```python
from build123d import *

# Parameters (mm, degrees)
SKETCH1_W               = 20.4
SKETCH1_H               = 17.7
SKETCH1_W_2             = 14.4
SKETCH1_H_2             = 11.7
SKETCH1_R               = 3.15
BOSS_EXTRUDE1_DEPTH     = 25
SKETCH1_3_W             = 20.4
SKETCH1_3_H             = 17.7
SKETCH1_3_W_2           = 14.4
SKETCH1_3_H_2           = 11.7
BOSS_EXTRUDE2_DEPTH     = 30
SKETCH2_W               = 22.449827962
SKETCH2_H               = 3
CUT_EXTRUDE1_DEPTH      = 15
FILLET1_R               = 10
SKETCH3_W               = 50
SKETCH3_H               = 20
SKETCH3_R               = 3.15
BOSS_EXTRUDE3_DEPTH     = 3
SKETCH4_R               = 1.7
CUT_EXTRUDE2_DEPTH      = 39.13135193
BOSS_EXTRUDE4_DEPTH     = 3
BOSS_EXTRUDE5_DEPTH     = 3
CHAMFER1_SIZE           = 3
CHAMFER2_SIZE           = 1
FILLET3_R               = 2
SKETCH7_W               = 14.4
SKETCH7_H               = 3
CUT_EXTRUDE3_DEPTH      = 5
BOSS_EXTRUDE6_DEPTH     = 5
CUT_EXTRUDE4_DEPTH      = 38.132499243
CUT_EXTRUDE4_DEPTH_BACK = 38.132499243
BOSS_EXTRUDE7_DEPTH     = 20.4


with BuildPart() as part:
    # Sketch1 → Boss-Extrude1 (new body)
    # profile 1 of 2: a face of its own
    with BuildSketch(Plane(origin=(0, 0, 0), x_dir=(1, 0, 0), z_dir=(0, 1, 0))):
        Rectangle(SKETCH1_W, SKETCH1_H)
        Rectangle(SKETCH1_W_2, SKETCH1_H_2, mode=Mode.SUBTRACT)
    # profile 2 of 2: a face of its own
    with BuildSketch(Plane(origin=(0, 0, 0), x_dir=(1, 0, 0), z_dir=(0, 1, 0))):
        Rectangle(SKETCH1_W_2, SKETCH1_H_2)
        with Locations(Location((0, 0, 0), (0, 0, 270))):
            Circle(SKETCH1_R, mode=Mode.SUBTRACT)
    extrude(amount=BOSS_EXTRUDE1_DEPTH)

    # Sketch1<3> → Boss-Extrude2 (add)
    with BuildSketch(Plane(origin=(0, 0, 0), x_dir=(1, 0, 0), z_dir=(0, 1, 0))):
        Rectangle(SKETCH1_3_W, SKETCH1_3_H)
        Rectangle(SKETCH1_3_W_2, SKETCH1_3_H_2, mode=Mode.SUBTRACT)
    extrude(amount=BOSS_EXTRUDE2_DEPTH)

    # Sketch2 → Cut-Extrude1 (cut)
    with BuildSketch(Plane(origin=(0, 30, 0), x_dir=(1, 0, 0), z_dir=(0, 1, 0))):
        with Locations((0, 8.85)):
            Rectangle(SKETCH2_W, SKETCH2_H)
    extrude(amount=-CUT_EXTRUDE1_DEPTH, mode=Mode.SUBTRACT)

    # Fillet1
    # the kernel refuses this fillet: 10 mm, written as the material it adds along each edge
    with BuildSketch(Plane(origin=(10.2, 15, -7.35), x_dir=(0, 1, 0), z_dir=(-1, 0, 0))) as fillet1_piece_1:
        with BuildLine():
            CenterArc((5.267826876, 10), FILLET1_R, 238.211669383, 31.788330617)
            Line((0, 1.5), (-0.105356538, 1.33))
            ThreePointArc((-0.105356538, 1.33), (-0.2, 0.75), (-0.2, 0))
            Line((-0.2, 0), (0, -0.2))
            Line((0, -0.2), (5.267826876, -0.2))
            Line((5.267826876, -0.2), (5.267826876, 0))
        make_face()
    extrude(amount=20.4)

    # Sketch3 → Boss-Extrude3 (add)
    with BuildSketch(Plane.XZ):
        Rectangle(SKETCH3_W, SKETCH3_H)
        with Locations(Location((0, 0, 0), (0, 0, 90))):
            Circle(SKETCH3_R, mode=Mode.SUBTRACT)
    extrude(amount=-BOSS_EXTRUDE3_DEPTH)

    # Sketch4 → Cut-Extrude2 (cut, through all)
    with BuildSketch(Plane(origin=(0, 3, 0), x_dir=(1, 0, 0), z_dir=(0, 1, 0))):
        with Locations(Location((-20, 0, 0), (0, 0, 270))):
            Circle(SKETCH4_R)
        with BuildLine():
            Line((18.4, 1.7), (20, 1.7))
            ThreePointArc((20, 1.7), (21.7, 0), (20, -1.7))
            Line((20, -1.7), (18.4, -1.7))
            ThreePointArc((18.4, -1.7), (16.7, 0), (18.4, 1.7))
        make_face()
    extrude(amount=-CUT_EXTRUDE2_DEPTH, mode=Mode.SUBTRACT)

    # Sketch5 → Boss-Extrude4 (add)
    with BuildSketch(Plane(origin=(0, 0, -8.85), x_dir=(-1, 0, 0), z_dir=(0, 0, -1))):
        Polygon((-10.2, 3), (-10.2, 9), (-12.2, 9), (-18.2, 3), align=None)
        Polygon((18.2, 3), (10.2, 3), (10.2, 9), (12.2, 9), align=None)
    extrude(amount=-BOSS_EXTRUDE4_DEPTH)

    # Sketch6 → Boss-Extrude5 (add)
    with BuildSketch(Plane.XY.offset(8.85)):
        Polygon((-18.2, 3), (-10.2, 3), (-10.2, 9), (-12.2, 9), align=None)
        Polygon((10.2, 9), (10.2, 3), (18.2, 3), (12.2, 9), align=None)
    extrude(amount=-BOSS_EXTRUDE5_DEPTH)

    # Chamfer1
    chamfer1_edges = [part.edges().sort_by_distance(p)[0] for p in [
        (-10.2, 3, 0),
        (10.2, 3, 0),
    ]]
    chamfer(chamfer1_edges, length=CHAMFER1_SIZE)

    # Chamfer2
    chamfer2_edges = [part.edges().sort_by_distance(p)[0] for p in [
        (0, 3, -8.85),
        (0, 3, 8.85),
    ]]
    chamfer(chamfer2_edges, length=CHAMFER2_SIZE)

    # Fillet3
    fillet3_edges = [part.edges().sort_by_distance(p)[0] for p in [
        (25, 1.5, 10),
        (25, 1.5, -10),
        (-25, 1.5, -10),
        (-25, 1.5, 10),
    ]]
    fillet(fillet3_edges, radius=FILLET3_R)

    # Sketch7 → Cut-Extrude3 (cut)
    with BuildSketch(Plane(origin=(0, 30, 0), x_dir=(1, 0, 0), z_dir=(0, 1, 0))):
        with Locations((0, -7.35)):
            Rectangle(SKETCH7_W, SKETCH7_H)
    extrude(amount=-CUT_EXTRUDE3_DEPTH, mode=Mode.SUBTRACT)

    # Sketch7<3> → Boss-Extrude6 (add)
    with BuildSketch(Plane(origin=(0, 30, 0), x_dir=(1, 0, 0), z_dir=(0, 1, 0))):
        Polygon((-7.2, -9.85), (-7.2, -8.85), (-10.2, -8.85), (-10.2, -11.35), (10.2, -11.35), (10.2, -8.85), (7.2, -8.85), (7.2, -9.85), align=None)
    extrude(amount=-BOSS_EXTRUDE6_DEPTH)

    # Sketch8 → Cut-Extrude4 (cut, two sides: drawn at the far end of the back side and taken through both)
    with BuildSketch(Plane(origin=(0, 25, 0), x_dir=(1, 0, 0), z_dir=(0, 1, 0)).offset(-CUT_EXTRUDE4_DEPTH_BACK)):
        with BuildLine():
            Line((3.15, 0), (3.15, -4))
            ThreePointArc((3.15, -4), (0, -7.15), (-3.15, -4))
            Line((-3.15, -4), (-3.15, 0))
            ThreePointArc((-3.15, 0), (0, 3.15), (3.15, 0))
        make_face()
    extrude(amount=CUT_EXTRUDE4_DEPTH + CUT_EXTRUDE4_DEPTH_BACK, mode=Mode.SUBTRACT)

    # Sketch9 → Boss-Extrude7 (add)
    with BuildSketch(Plane.ZY.offset(10.2)):
        Polygon((11.35, 25), (8.85, 25), (8.85, 15), align=None)
    extrude(amount=-BOSS_EXTRUDE7_DEPTH)


solid = part.part
```
Could you check a few things on this model? Use its own coordinates, in mm. A direction names the side the tool comes from. Round coordinates to 2 decimals unless told otherwise and drop trailing zeros. Order: outer loops, then holes, each group sorted by start corner. A loop starts at its lowest first (then second) coordinate and runs counter-clockwise, first axis right, second up. Notation, with made-up numbers: M -14,-6 L 14,-6 A5 ccw 14,-2 Z; hole C 41,-18.5 d4. An arc over 180 degrees is marked long. One line per question, with ' | ' between items. Start each with the question number.
(1) Thinking about a two-plate mould opening in X: for faces 5 (the face through (24.43, 1.52, -9.4)), 6 (the face through (0.07, 12.32, -3.15)), 7 (the face through (13, 5, 5.85)), which applies, +X half, -X half, draft (parallel to the pull), parting line (faces both ways), or undercut?
(2) Suppose I cut it at A-A on x = 0. List the corners of the cut face in (y, z) for me.
(3) Suppose I cut it at B-B on y = 11.5. List the corners of the cut face in (x, z) for me.
(4) Suppose I cut it at D-D on x = -20. List the corners of the cut face in (y, z) for me, then the cut area to 3 significant figures.
(5) Please list where these lines run through material, in increasing order: line 1 along X through (y, z) = (10, 2.75); line 2 along Y through (x, z) = (-16, -0.75).
(6) For faces 1 (the face through (0.07, 12.32, 7.15)), 2 (the face through (-11, 9, -7)), 3 (the face through (-11.7, 4.5, 0.1)), 4 (the face through (11, 9, -7)), which set-ups out of +Z, -Z, +X, -X, +Y, -Y let a thin tool reach every point of the face, with its end or its side?
(7) Suppose I cut it at C-C on z = 2.25. List the corners of the cut face in (x, y) for me, then the cut area to 3 significant figures.
(8) For P1, Ø3, axis at x = 2, z = 8, coming from the +Y side; P2, Ø1.2, axis at y = 17.5, z = 2.5, coming from the -X side; P3, Ø1.8, axis at x = 19, y = 1, coming from the +Z side, each with a flat end and sliding along its axis, tell me the tip position at first contact or that it passes through.
Geometry results:
1) face 5: +X half | face 6: undercut | face 7: draft
2) outline: M 0,-10 L 3,-10 L 3,-9.85 L 4,-8.85 L 15,-8.85 A10 cw 20.27,-7.35 L 30,-7.35 L 30,-5.85 L 25,-5.85 L 25,-3.15 L 0,-3.15 Z; M 0,7.15 L 25,7.15 L 25,9.85 L 30,9.85 L 30,11.35 L 25,11.35 L 15,8.85 L 4,8.85 L 3,9.85 L 3,10 L 0,10 Z
3) outline: M -10.2,-8.85 L 10.2,-8.85 L 10.2,8.85 L -10.2,8.85 Z; hole M -3.15,0 A3.15 ccw 3.15,0 L 3.15,4 A3.15 ccw -3.15,4 Z
4) outline: M 0,-10 L 3,-10 L 3,-1.7 L 0,-1.7 Z; M 0,1.7 L 3,1.7 L 3,10 L 0,10 Z | area: 49.8 mm²
5) line 1: -10.2 to -3.15, 3.15 to 10.2 | line 2: 0 to 3
6) face 1: +Y, -Y | face 2: +Z, -Z, -X, +Y | face 3: -X, +Y | face 4: +Z, -Z, +X, +Y
7) outline: M -25,0 L -3.15,0 L -3.15,25 L -7.2,25 L -7.2,30 L -10.2,30 L -10.2,6 L -13.2,3 L -25,3 Z; M 3.15,0 L 25,0 L 25,3 L 13.2,3 L 10.2,6 L 10.2,30 L 7.2,30 L 7.2,25 L 3.15,25 Z | area: 480 mm²
8) P1: y = 25 | P2: x = -10.2 | P3: z = 10
